Study the drawing (mm; zero at the part's minimum x, y, z) and answer. A direction names the side the tool comes from. Give positions to 0.01 mm unless a question says otherwise; leave off trailing zeros. Write each loop counter-clockwise with the first axis right and the second up, starting at its lowest first coordinate (ties: lowest second). Pieces come first, ordered by that corner, then holes. Notation, with made-up numbers: (-8.75, -0.75) - (24.25, -0.75) arc R18 ccw to (24.25, 19.25) - close; hole circle Ø5 at (88, 14). An arc over 180 degrees is marked (long way). Answer as CSV lines item,"result".
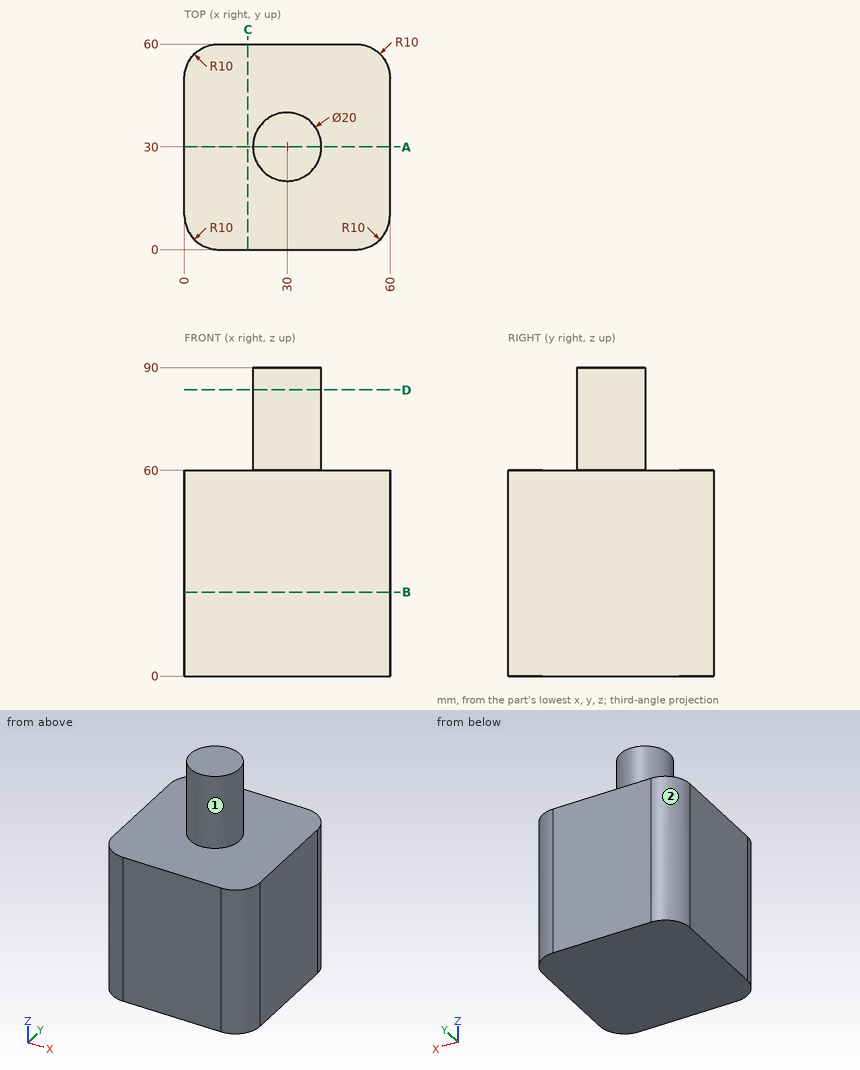
(1) This flat-tipped pin is pushed along its axis until it touches: P1, Ø4, axis at x = 28, y = 49, coming from the +Z side. Where does it stop, or does it pass through?
Worked out:
P1,"stops at z = 60"
(2) A cutting plane is placed at D-D (z = 83.5). Write down the section's boundary in (x, y).
Worked out:
outline,"circle Ø20 at (30, 30)"
(3) Find the intervals of material crossed by L1, parallel to Z at x = 50.5, y = 44.5; L2, parallel to X at y = 29.5, z = 72.5; L3, parallel to Y at x = 8.5, z = 41, in increasing order.
Worked out:
L1,"z = 0 to 60"
L2,"x = 20.01 to 39.99"
L3,"y = 0.11 to 59.89"
(4) A cutting plane is placed at C-C (x = 18.5). Write down the section's boundary in (y, z), and give its area (3 significant figures).
Worked out:
outline,"(0, 0) - (60, 0) - (60, 60) - (0, 60) - close"
area,"3,600 mm^2"
(5) For the marked faces 1 and 2, determine the directions among +Z, -Z, +X, -X, +Y, -Y from which every point of the face is accessible in a straight line to the end or side of a thin tool.
Worked out:
face 1,"+Z"
face 2,"+Z, -Z, -X, +Y"
(6) A cutting plane is placed at A-A (y = 30). Write down the section's boundary in (x, z).
Worked out:
outline,"(0, 0) - (60, 0) - (60, 60) - (40, 60) - (40, 90) - (20, 90) - (20, 60) - (0, 60) - close"
(7) A cutting plane is placed at B-B (z = 24.5). Write down the section's boundary in (x, y), and give its area (3 significant figures).
Worked out:
outline,"(0, 10) arc R10 ccw to (10, 0) - (50, 0) arc R10 ccw to (60, 10) - (60, 50) arc R10 ccw to (50, 60) - (10, 60) arc R10 ccw to (0, 50) - close"
area,"3,510 mm^2"
